```python
from build123d import *

# Parameters (mm, degrees)
BOSS_EXTRUDE1_DEPTH = 26.4
SKETCH2_R           = 1.75
CUT_EXTRUDE1_DEPTH  = 40.842252323
CUT_EXTRUDE3_START  = -10
CUT_EXTRUDE3_DEPTH  = 30.842252323
BOSS_EXTRUDE2_DEPTH = 10


with BuildPart() as part:
    # Sketch1 → Boss-Extrude1 (new body)
    with BuildSketch(Plane(origin=(0, 0, 0), x_dir=(1, 0, 0), z_dir=(0, 1, 0))):
        with BuildLine():
            Line((0, 23.60895106), (0, -23.60895106))
            Line((0, -23.60895106), (18.25, -23.60895106))
            Line((18.25, -23.60895106), (18.25, -14.10895106))
            ThreePointArc((18.25, -14.10895106), (6, 0), (18.25, 14.10895106))
            Line((18.25, 14.10895106), (18.25, 23.60895106))
            Line((18.25, 23.60895106), (0, 23.60895106))
        make_face()
    extrude(amount=BOSS_EXTRUDE1_DEPTH)

    # Sketch2 → Cut-Extrude1 (cut, through all)
    with BuildSketch(Plane(origin=(18.25, 0, 0), x_dir=(0, 0, -1), z_dir=(1, 0, 0))):
        with Locations((-18.85895106, 13.2)):
            Circle(SKETCH2_R)
    cut_extrude1 = extrude(amount=-CUT_EXTRUDE1_DEPTH, mode=Mode.SUBTRACT)

    # Sketch5 → Cut-Extrude3 (cut, through all)
    with BuildSketch(Plane(origin=(18.25, 0, 0), x_dir=(0, 0, -1), z_dir=(1, 0, 0)).offset(CUT_EXTRUDE3_START)):
        Polygon((-17.242370306, 16), (-20.475531813, 16), (-22.092112567, 13.2), (-20.475531813, 10.4), (-17.242370306, 10.4), (-15.625789552, 13.2), align=None)
    cut_extrude3 = extrude(amount=-CUT_EXTRUDE3_DEPTH, mode=Mode.SUBTRACT)

    # Mirror1: Cut-Extrude1, Cut-Extrude3 across plane
    add(cut_extrude1.mirror(Plane.XY), mode=Mode.SUBTRACT)
    add(cut_extrude3.mirror(Plane.XY), mode=Mode.SUBTRACT)

    # Sketch7 → Boss-Extrude2 (add, symmetric)
    with BuildSketch(Plane.XY):
        Polygon((0, 0), (-8.957359313, 0), (-36.415999231, -27.458639918), (-42.921381618, -20.953257531), (-36.557420587, -14.589296501), (-34.436100244, -16.710616844), (-38.678740931, -20.953257531), (-36.415999231, -23.215999231), (0, 13.2), (-36.415999231, 49.615999231), (-38.678740931, 47.353257531), (-34.436100244, 43.110616844), (-36.557420587, 40.989296501), (-42.921381618, 47.353257531), (-36.415999231, 53.858639918), (-8.957359313, 26.4), (0, 26.4), (6, 26.4), (6, 0), align=None)
    extrude(amount=BOSS_EXTRUDE2_DEPTH, both=True)


solid = part.part
```
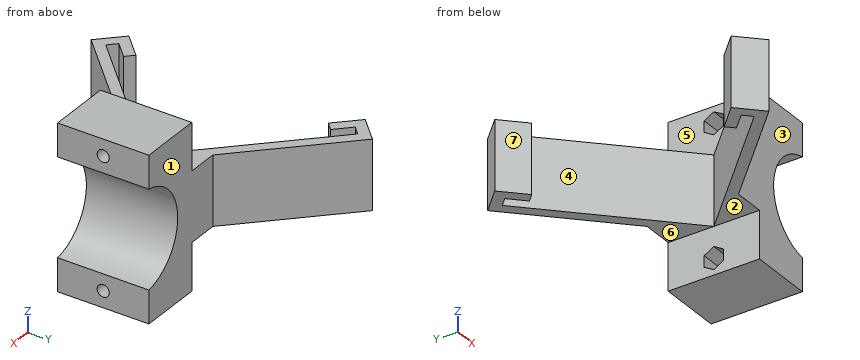
Input: part model. Units: mm. Frame: model coordinates. Face numbers are marked on the shaded views. A direction names the side the tool comes from. Give positions to 0.01 mm unless a question says otherwise; leave off trailing zeros. Write each loop counter-clockwise with the first axis right and the second up, starting at its lowest first coordinate (ties: lowest second). Pieces come first, ordered by that corner, then holes. Notation, with made-up numbers: (-6, -34.5) - (17, -34.5) arc R22 cw to (17, -16.5) - close; hole circle Ø6 at (63, -30.5). An arc over 180 degrees is marked (long way). Write item = value, one per line. Start each with the question number.
1. Section query A-A, the plane x = -20.5. Output: boundary loops of the cut face in (y, z).
2. Section query C-C, the plane x = 3. Output: boundary loops of the cut face in (y, z), then the cut area to 3 significant figures.
3. Ray query, L1, parallel to Y at x = -36.5, z = 9; L2, parallel to Y at x = -35.5, z = -2; L3, parallel to Z at x = 14, y = 13. Return the intervals inside material, ascending.
4. Section query B-B, the plane y = 23. Output: boundary loops of the cut face in (x, z), then the cut area to 3 significant figures.
5. Section query D-D, the plane z = -19. Output: boundary loops of the cut face in (x, y).
6. First-contact query: pin 1 Ø8 at (x, z) = (5, 4) entering from +Y; pin 2 Ø4 at (x, y) = (-8.5, 27.5) entering from -Z; pin 3 Ø6 at (x, z) = (-9, 11.5) entering from +Y; pin 4 Ø12 at (x, y) = (-27.5, -0.5) entering from -Z. Flat tips, straight axial feed; report the tip coordinate or a pass-through.
7. Mould query, pull axis Y, two halves, no side actions, for the marked faces 1, 2, 3 and 4. Classes: released by +Y, released by -Y, zero draft, split by the parting line, or undercut.
8. Access query for the marked faces 5, 6 and 7. Directions: +Z, -Z, +X, -X, +Y, -Y. A direction counts if a zero-diameter tool reaches every point of the face in a straight line with its end or side. Return the directions, or none.
Check sheet entries:
q1.outline = (-11.54, -10) - (-7.3, -10) - (-7.3, 10) - (-11.54, 10) - close; (33.7, -10) - (37.94, -10) - (37.94, 10) - (33.7, 10) - close
q2.outline = (0, -23.61) - (26.4, -23.61) - (26.4, 23.61) - (0, 23.61) - close; hole (10.4, -20.48) - (13.2, -22.09) - (16, -20.48) - (16, -17.24) - (13.2, -15.63) - (10.4, -17.24) - close; hole (10.4, 17.24) - (13.2, 15.63) - (16, 17.24) - (16, 20.48) - (13.2, 22.09) - (10.4, 20.48) - close
q2.area = 1,190 mm2
q3.L1 = -27.37 to -23.13, -18.77 to -14.65, 41.05 to 45.17, 49.53 to 53.77
q3.L2 = -26.54 to -22.3, -17.77 to -15.65, 42.05 to 44.17, 48.7 to 52.94
q3.L3 = -23.61 to -20.6, -17.12 to -12.81, 12.81 to 17.12, 20.6 to 23.61
q4.outline = (-9.8, -10) - (0, -10) - (0, -23.61) - (18.25, -23.61) - (18.25, -14.11) arc R14.25 cw to (18.25, 14.11) - (18.25, 23.61) - (0, 23.61) - (0, 10) - (-9.8, 10) - close
q4.area = 796 mm2
q5.outline = (0, 0) - (18.25, 0) - (18.25, 11.46) - (8.25, 11.46) - (8.25, 10.4) - (0, 10.4) - close; (0, 16) - (8.25, 16) - (8.25, 14.94) - (18.25, 14.94) - (18.25, 26.4) - (0, 26.4) - close
q6.pin_1 = 26.4
q6.pin_2 = -10
q6.pin_3 = 29.04
q6.pin_4 = through
q7.face_1 = released by +Y
q7.face_2 = zero draft
q7.face_3 = released by -Y
q7.face_4 = undercut
q8.face_5 = +Z, -X, +Y, -Y
q8.face_6 = -Z, -X, +Y, -Y
q8.face_7 = +Z, -Z, -X
